from build123d import *

# Parameters (mm, degrees)
SKETCH_1_W           = 15
SKETCH_1_H           = 14.5
EXTRUDE_1_DEPTH      = 12.85
EXTRUDE_2_DEPTH      = 3.3
EXTRUDE_2_DEPTH_BACK = 1
SKETCH_2_R           = 1.18
CUT_EXTRUDE_1_DEPTH  = 10


with BuildPart() as part:
    # 草图1 → 凸台-拉伸1 (new body)
    with BuildSketch(Plane(origin=(0, 0, 0), x_dir=(1, 0, 0), z_dir=(0, 1, 0))):
        Rectangle(SKETCH_1_W, SKETCH_1_H)
    extrude(amount=EXTRUDE_1_DEPTH)

    # 草图2 → 凸台-拉伸2 (add, two sides: drawn at the far end of the back side and taken through both)
    with BuildSketch(Plane.XZ.offset(-EXTRUDE_2_DEPTH_BACK)):
        with Locations(Location((-7.5, 0, 0), (0, 0, 270))):
            Circle(SKETCH_2_R)
        with Locations(Location((7.5, 0, 0), (0, 0, 90))):
            Circle(SKETCH_2_R)
    extrude(amount=EXTRUDE_2_DEPTH + EXTRUDE_2_DEPTH_BACK)

    # 草图3 → 切除-拉伸1 (cut)
    with BuildSketch(Plane.XY.offset(7.25)):
        Polygon((2.967608293, 11.336409161), (-2.967608293, 11.336409161), (-2.967608293, 9.376154142), (-4.383348029, 9.376154142), (-4.383348029, 7.688156764), (-6.615860689, 7.688156764), (-6.615860689, 1.807391707), (6.615860689, 1.807391707), (6.615860689, 7.688156764), (4.383348029, 7.688156764), (4.383348029, 9.376154142), (2.967608293, 9.376154142), align=None)
    extrude(amount=-CUT_EXTRUDE_1_DEPTH, mode=Mode.SUBTRACT)


solid = part.part
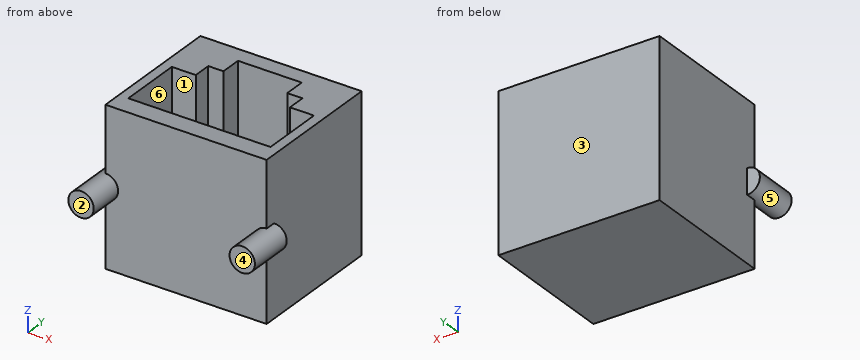
Could you check a few things on this model? Use its own coordinates, in mm. Face numbers are marked on the shaded views. A direction names the side the tool comes from. Round coordinates to 2 decimals unless told otherwise and drop trailing zeros. Write each loop counter-clockwise with the first axis right and the second up, starting at its lowest first coordinate (ties: lowest second). Pieces come first, ordered by that corner, then holes. Notation, with made-up numbers: (63, -29.5) - (94, -29.5) arc R14 cw to (94, -6.5) - close; hole circle Ø11 at (7, 50.25). An arc over 180 degrees is marked (long way). Use a Markdown table: item, result.
Q1. Thinking about a two-plate mould opening in Y: for the marked faces 1, 2 and 3, which applies, released by +Y, released by -Y, zero draft, split by the parting line, or undercut?
Output values:
| item | result |
|---|---|
| face 1 | undercut |
| face 2 | released by -Y |
| face 3 | released by +Y |
Q2. Please list where these lines run through material, in increasing order: L1, parallel to Y at x = -1, z = 3; L2, parallel to X at y = 9, z = 4; L3, parallel to Y at x = 5.75, z = 6.25.
Output values:
| item | result |
|---|---|
| L1 | 0 to 1.81, 11.34 to 12.85 |
| L2 | -7.5 to -4.38, 4.38 to 7.5 |
| L3 | 0 to 1.81, 7.69 to 12.85 |
Q3. I want a section at C-C (x = -0.5). List the corners of the cut face in (y, z) for me, plus the area to 3 significant figures.
Output values:
| item | result |
|---|---|
| outline | (0, -7.25) - (12.85, -7.25) - (12.85, 7.25) - (11.34, 7.25) - (11.34, -2.75) - (1.81, -2.75) - (1.81, 7.25) - (0, 7.25) - close |
| area | 91.0 mm2 |
Q4. For pin 1 (1.8 mm diameter, centred on y = 5.5, z = 3, fed in from -X); pin 2 (0.8 mm diameter, centred on y = 9, z = 4.5, fed in from +X); pin 3 (2 mm diameter, centred on x = 6, z = -3.5, fed in from -Y); pin 4 (1.3 mm diameter, centred on x = -8, z = 0.5, fed in from +Y), each with a flat end and sliding along its axis, tell me the tip position at first contact or that it passes through.
Output values:
| item | result |
|---|---|
| pin 1 | x = -7.5 |
| pin 2 | x = 7.5 |
| pin 3 | y = 0 |
| pin 4 | y = 12.85 |
Q5. I want a section at B-B (y = 7.25). List the corners of the cut face in (x, z) for me.
Output values:
| item | result |
|---|---|
| outline | (-7.5, -7.25) - (7.5, -7.25) - (7.5, 7.25) - (6.62, 7.25) - (6.62, -2.75) - (-6.62, -2.75) - (-6.62, 7.25) - (-7.5, 7.25) - close |
Q6. For the marked faces 4, 5 and 6, which set-ups out of +Z, -Z, +X, -X, +Y, -Y let a thin tool reach every point of the face, with its end or its side?
Output values:
| item | result |
|---|---|
| face 4 | +Z, -Z, +X, -X, -Y |
| face 5 | -Y |
| face 6 | +Z |
Q7. I want a section at A-A (z = -2.5). List the corners of the cut face in (x, y) for me, plus the area to 3 significant figures.
Output values:
| item | result |
|---|---|
| outline | (-7.5, 0) - (7.5, 0) - (7.5, 12.85) - (-7.5, 12.85) - close; hole (-6.62, 1.81) - (6.62, 1.81) - (6.62, 7.69) - (4.38, 7.69) - (4.38, 9.38) - (2.97, 9.38) - (2.97, 11.34) - (-2.97, 11.34) - (-2.97, 9.38) - (-4.38, 9.38) - (-4.38, 7.69) - (-6.62, 7.69) - close |
| area | 88.5 mm2 |
Q8. I want a section at D-D (z = 0). List the corners of the cut face in (x, y) for me.
Output values:
| item | result |
|---|---|
| outline | (-8.68, -3.3) - (-6.32, -3.3) - (-6.32, 0) - (6.32, 0) - (6.32, -3.3) - (8.68, -3.3) - (8.68, 1) - (7.5, 1) - (7.5, 12.85) - (-7.5, 12.85) - (-7.5, 1) - (-8.68, 1) - close; hole (-6.62, 1.81) - (6.62, 1.81) - (6.62, 7.69) - (4.38, 7.69) - (4.38, 9.38) - (2.97, 9.38) - (2.97, 11.34) - (-2.97, 11.34) - (-2.97, 9.38) - (-4.38, 9.38) - (-4.38, 7.69) - (-6.62, 7.69) - close |
